Input: part model. Units: mm. Frame: model coordinates. A direction names the side the tool comes from. Coordinates: 2 decimals unless noted, no trailing zeros. Order: outer loops, then holes, each group sorted by start corner. A loop starts at its lowest first (then second) coordinate and runs counter-clockwise, first axis right, second up. Notation, with made-up numbers: (28.25, 7) -> (40.25, 7) arc R35 cw to (40.25, 45) -> close; hole circle Ø3 at (-14.5, 84). An arc over 180 degrees is marked (long way). Answer as CSV lines item,"result".
from build123d import *

# Parameters (mm, degrees)
F1_DEPTH = 8
F2_R     = 3.1
F3_DEPTH = 8
F4_R     = 3
F5_DEPTH = 16


with BuildPart() as f1:
    # F0 (on Front) → F1 (new body)
    with BuildSketch(Plane.XZ):
        Polygon((-80, -10.675645), (-80, 14.487543), (-88, 14.487543), (-88, -18.675645), (0, -18.675645), (0, -10.675645), align=None)
    extrude(amount=F1_DEPTH)

    # F2 (on Right) → F3 (join)
    with BuildSketch(Plane.YZ):
        with Locations((-4.106534, -14.342085)):
            Circle(F2_R)
    extrude(amount=F3_DEPTH)

    # F4 (on Top) → F5 (cut)
    with BuildSketch(Plane.XY):
        with Locations((-83.8, -3.8)):
            Circle(F4_R)
    extrude(amount=F5_DEPTH, mode=Mode.SUBTRACT)


solid = f1.part
1. Mould query, pull axis Y, two halves, no side actions, for faces 4 (the face through (3.94, -4.78, -17.37)), 5 (the face through (-84, -4, 0)), 6 (the face through (-54, -8, -12)). Classes: released by +Y, released by -Y, zero draft, split by the parting line, or undercut.
Findings:
face 4,"split by the parting line"
face 5,"undercut"
face 6,"released by -Y"
2. Cut plane C-C (y = -3.8). Return the cut outline in (x, z), plus the area to 3 significant figures.
Findings:
outline,"(-88, -18.68) -> (0, -18.68) -> (0, -17.43) -> (8, -17.43) -> (8, -11.26) -> (0, -11.26) -> (0, -10.68) -> (-80, -10.68) -> (-80, 14.49) -> (-80.8, 14.49) -> (-80.8, 0) -> (-86.8, 0) -> (-86.8, 14.49) -> (-88, 14.49) -> close"
area,"868 mm2"
3. Cut plane B-B (x = -83.8). Return the cut outline in (y, z), plus the area to 3 significant figures.
Findings:
outline,"(-8, -18.68) -> (0, -18.68) -> (0, 14.49) -> (-0.8, 14.49) -> (-0.8, 0) -> (-6.8, 0) -> (-6.8, 14.49) -> (-8, 14.49) -> close"
area,"178 mm2"
4. Contact query for flat-ended pins moving along their axis: pin 1 (4 mm diameter, centred on y = -4.5, z = -3, fed in from +X); pin 2 (4 mm diameter, centred on x = -35.5, y = -5, fed in from +Z). Output: stop coordinate, or through.
Findings:
pin 1,"stops at x = -80"
pin 2,"stops at z = -10.68"
5. Cut plane D-D (z = -7.5). Return the cut outline in (x, y), plus the area to 3 significant figures.
Findings:
outline,"(-88, -8) -> (-80, -8) -> (-80, 0) -> (-88, 0) -> close"
area,"64.0 mm2"
6. Cut plane A-A (z = 4). Return the cut outline in (x, y), plus the area to 3 significant figures.
Findings:
outline,"(-88, -8) -> (-80, -8) -> (-80, 0) -> (-88, 0) -> close; hole circle Ø6 at (-83.8, -3.8)"
area,"35.7 mm2"
7. Reachability of faces 1 (the face through (-86.2, -5.6, 7.1)), 2 (the face through (-39, -4, -10.676)), 3 (the face through (0, -1, -16)) from +Z, -Z, +X, -X, +Y, -Y: full face, straight path, thin tool, end or side. Return the list, or none.
Findings:
face 1,"+Z"
face 2,"+Z, +X, +Y, -Y"
face 3,"+X"
8. Ray query, line 1 along Y through (x, z) = (-83.8, 8.75); line 2 along X through (y, z) = (-3.8, 5); line 3 along Z through (x, y) = (-67.5, -6.25). Return the intervals inside material, ascending.
Findings:
line 1,"y = -8 to -6.8, -0.8 to 0"
line 2,"x = -88 to -86.8, -80.8 to -80"
line 3,"z = -18.68 to -10.68"
